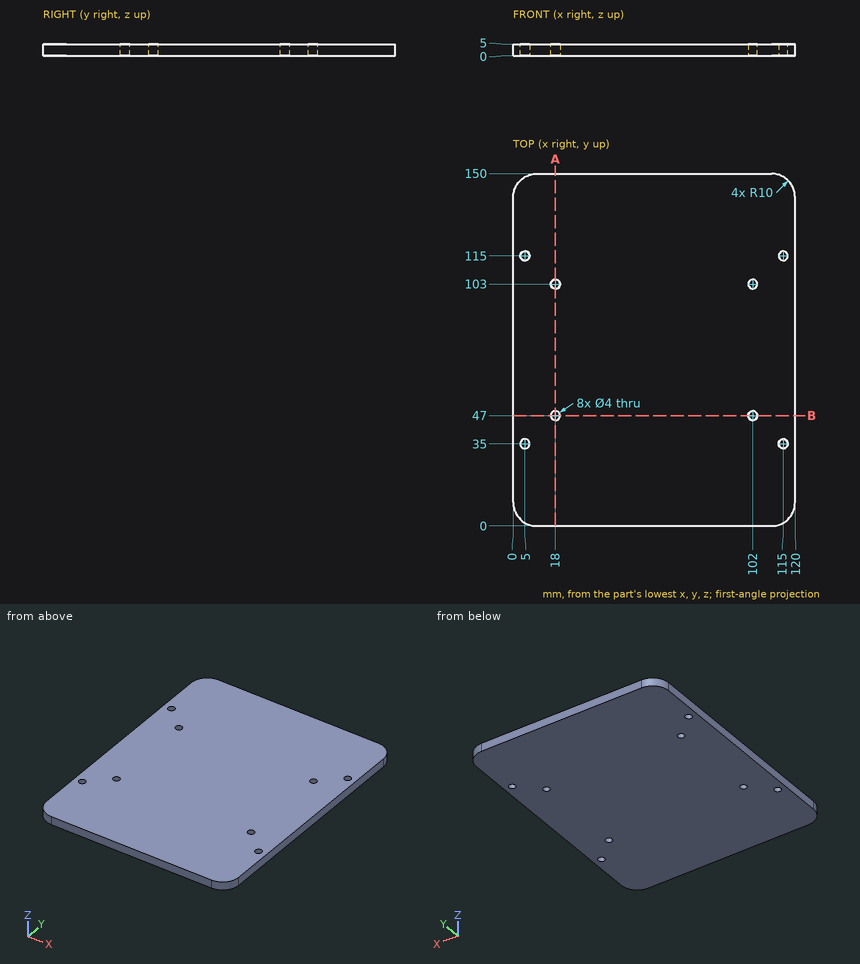
The figure shows three views and two pictorial views of one solid part (mm, origin at its lowest corner). Answer the questions. Give positions to 0.01 mm unless a question says otherwise; leave off trailing zeros. Write each loop counter-clockwise with the first axis right and the second up, starting at its lowest first coordinate (ties: lowest second). Pieces come first, ordered by that corner, then holes.
Q1. Straight lines are drawn through the part: L1, parallel to X at y = 103, z = 1.6; L2, parallel to Y at x = 102, z = 3.6; L3, parallel to X at y = 115, z = 1.95. For each, find the intervals that lie inside material, in ascending order.
Answer:
L1: x = 0 to 16, 20 to 100, 104 to 120
L2: y = 0 to 45, 49 to 101, 105 to 150
L3: x = 0 to 3, 7 to 113, 117 to 120
Q2. The part is cut by section A-A on x = 18. Give the vertices of the cut face in (y, z).
Answer:
outline: (0, 0) - (45, 0) - (45, 5) - (0, 5) - close; (49, 0) - (101, 0) - (101, 5) - (49, 5) - close; (105, 0) - (150, 0) - (150, 5) - (105, 5) - close
Q3. Given pin 1 (4.5 mm diameter, centred on x = 18, y = 47, fed in from +Z); pin 2 (3 mm diameter, centred on x = 102, y = 103, fed in from +Z), each flat-ended and moving along its own axis, determine where each tip first touches the part or whether it passes through.
Answer:
pin 1: stops at z = 5
pin 2: passes through
Q4. The part is cut by section B-B on y = 47. Give the vertices of the cut face in (x, z).
Answer:
outline: (0, 0) - (16, 0) - (16, 5) - (0, 5) - close; (20, 0) - (100, 0) - (100, 5) - (20, 5) - close; (104, 0) - (120, 0) - (120, 5) - (104, 5) - close
